Autodesk Inventor part; units mm, degrees
ref_plane "YZ Plane" through (0, 0, 0) normal (1, 0, 0) x (0, 1, 0)
ref_plane "XZ Plane" through (0, 0, 0) normal (0, 1, 0) x (-1, 0, 0)
ref_plane "XY Plane" through (0, 0, 0) normal (0, 0, 1) x (1, 0, 0)
sketch "Sketch1" plane through (0, 0, 0) normal (0, 0, 1) x (1, 0, 0)
  circle A0 centre (0, 0) radius 2.5
  dimension "d0" = 5
sketch "Sketch3" plane through (0, 0, 0) normal (1, 0, 0) x (0, 1, 0)
  line L0 (0, 0) -> (0, -13.011)
  line L1 (3.3076, -19.2298) -> (41.1924, -44.7702)
  line L2 (44.5, -50.989) -> (44.5, -67)
  arc A0 (0, -13.011) -> (3.3076, -19.2298) centre (7.5, -13.011) ccw
  arc A1 (44.5, -50.989) -> (41.1924, -44.7702) centre (37, -50.989) ccw
  point P0 (0, -17)
  point P1 (44.5, -47)
  dimension "d1" = 17
  dimension "d2" = 30
  dimension "d3" = 44.5
  dimension "d4" = 20
  dimension "d5" = 7.5
sweep "Sweep1" add profiles "Sketch1" path "Sketch3"
shell "Shell1" thickness 0.5 removed faces 2 at (1.2757, -0.3919, 0) at (0.6238, 43.9474, -67)
properties part number "158" material "Iron, Gray"
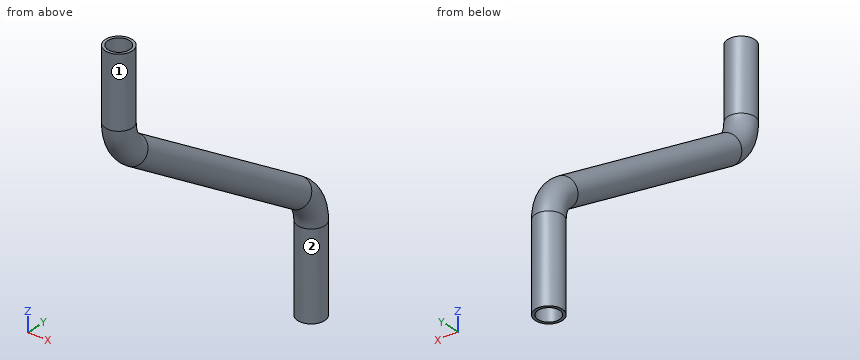
Geometry check sheet. Reference: the model listing, model coordinates, mm. Face numbers are marked on the shaded views. A direction names the side the tool comes from. Give positions to 0.01 mm unless a question says otherwise; leave off trailing zeros. Loops run counter-clockwise (first coordinate to the right, second up) from the corner with the lowest first, then second, coordinate; pieces in that order, holes last. Notation, with made-up numbers: (-20, 69) -> (-8, 69) arc R25 ccw to (-8, 89) -> close; hole circle Ø8 at (15.25, -25.5). An arc over 180 degrees is marked (long way). Answer in a Markdown table with one row per item. Add a question column.
1) Cross-section at A-A on z = -61. Record the boundary of the cut face in (x, y), and give its area (3 significant figures).
2) Gauge pin test, flat ends, axial feed: P1, Ø2, axis at x = 1, z = -24.5, coming from the +Y side; P2, Ø2.5, axis at x = 0, y = 44.5, coming from the +Z side; P3, Ø1.5, axis at x = 0, z = -42.5, coming from the -Y side. Record the tip position at first contact, or that the pin passes through.
3) Set-up check for the marked faces 1 and 2: record each of +Z, -Z, +X, -X, +Y, -Y from which the full face is reachable in a straight line by a thin tool's end or side.
4) Material ranges on probe 1 along Y at (x, z) = (0, -5.75); probe 2 along Y at (x, z) = (0, -55.5), recorded low to high. Write a range as from..to.
Outcome:
| question | item | result |
|---|---|---|
| 1 | outline | circle Ø5 at (0, 44.5); hole circle Ø4 at (0, 44.5) |
| 1 | area | 7.07 mm^2 |
| 2 | P1 | stops at y = 16.83 |
| 2 | P2 | stops at z = -43.18 |
| 2 | P3 | stops at y = 32.24 |
| 3 | face 1 | +Z |
| 3 | face 2 | -Z |
| 4 | probe 1 | y = -2.5..-2, 2..2.5 |
| 4 | probe 2 | y = 42..42.5, 46.5..47 |
